```python
from build123d import *

# Parameters (mm, degrees)
SKETCH_1_W               = 362
SKETCH_1_H               = 68
SM_BASE_FLANGE_1_DEPTH   = 1.5
SKETCH_6_R               = 2.5
CUT_EXTRUDE_1_DEPTH      = 10
SKETCH_7_W               = 40
SKETCH_7_H               = 42
SM_BASE_FLANGE_1_2_DEPTH = 1.5
SM_EDGE_FLANGE_1_DEPTH   = 422


# Sheet-metal steps are written as plain solids
with BuildPart() as part:
    # Sketch 1 → Sm Base Flange 1 (new body)
    with BuildSketch(Plane(origin=(0, 0, 0), x_dir=(0, 0, -1), z_dir=(1, 0, 0))):
        with Locations((0, -34)):
            Rectangle(SKETCH_1_W, SKETCH_1_H)
    extrude(amount=-SM_BASE_FLANGE_1_DEPTH)

    # Эскиз6 → Вырез-Вытянуть1 (cut)
    with BuildSketch(Plane(origin=(0, 0, 0), x_dir=(0, 0, -1), z_dir=(1, 0, 0))):
        with Locations((158, -10)):
            Circle(SKETCH_6_R)
        with Locations((128, -10)):
            Circle(SKETCH_6_R)
        with Locations(Location((-128, -10, 0), (0, 0, 180))):
            Circle(SKETCH_6_R)
        with Locations(Location((-158, -10, 0), (0, 0, 180))):
            Circle(SKETCH_6_R)
    extrude(amount=-CUT_EXTRUDE_1_DEPTH, mode=Mode.SUBTRACT)

    # Эскиз7 → Sm Base Flange 1 2 (add)
    with BuildSketch(Plane(origin=(0, 0, 0), x_dir=(0, 0, -1), z_dir=(1, 0, 0))):
        with Locations((-201, -21)):
            Rectangle(SKETCH_7_W, SKETCH_7_H)
        with Locations((201, -21)):
            Rectangle(SKETCH_7_W, SKETCH_7_H)
    extrude(amount=-SM_BASE_FLANGE_1_2_DEPTH)

    # Ребро-кромка1 section (across the edge) → Ребро-кромка1 (add)
    with BuildSketch(Plane(origin=(0, 1.5, -211), x_dir=(0, -1, 0), z_dir=(0, 0, 1))):
        with BuildLine():
            Line((-1.5, 1.5), (-1.5, 12))
            Line((-1.5, 12), (0, 12))
            Line((0, 12), (0, 1.5))
            ThreePointArc((0, 1.5), (0.439339828, 0.439339828), (1.5, 0))
            Line((1.5, 0), (1.5, -1.5))
            ThreePointArc((1.5, -1.5), (-0.621320344, -0.621320344), (-1.5, 1.5))
        make_face()
    extrude(amount=SM_EDGE_FLANGE_1_DEPTH)


solid = part.part
```
Verification items for the finished model (mm, model axes). A direction names the side the tool comes from. Give positions to 0.01 mm unless a question says otherwise; leave off trailing zeros. Loops run counter-clockwise (first coordinate to the right, second up) from the corner with the lowest first, then second, coordinate; pieces in that order, holes last. Notation, with made-up numbers: M 41,14 L 84,14 A7 ccw 84,24 Z; hole C -21,-39.5 d3. An arc over 180 degrees is marked long. One line per question, with ' | ' between items.
Item 1: Section check B-B, the plane y = -46.5. Record the cut outline in (x, z), plus the area to 3 significant figures.
Completed:
outline: M -1.5,-181 L 0,-181 L 0,181 L -1.5,181 Z | area: 543 mm^2
Item 2: Thickness scan on line 1 (Y direction, x = -1.05, z = -158); line 2 (X direction, y = -7, z = -16); line 3 (Y direction, x = 8.5, z = 94). Record the ranges inside material, lowest first. Write a range as [from, to].
Completed:
line 1: y = [-68, -12.5], [-7.5, 1.58] | line 2: x = [-1.5, 0] | line 3: y = [1.5, 3]
Item 3: Depth check by flat-ended pin: P1, Ø0.8, axis at x = -1, z = 214, coming from the +Y side; P2, Ø1.6, axis at x = -0.5, z = -195.5, coming from the -Y side; P3, Ø8, axis at x = 3.5, y = -59, coming from the -Z side; P4, Ø0.9, axis at x = 2, y = 1, coming from the -Z side. Enter the tip coordinate at first touch or a pass-through.
Completed:
P1: stops at y = 0 | P2: stops at y = -42 | P3: stops at z = -181 | P4: passes through
Item 4: Section check A-A, the plane z = -104. Record the cut outline in (x, y).
Completed:
outline: M -1.5,-68 L 0,-68 L 0,0 A1.5 cw 1.5,1.5 L 12,1.5 L 12,3 L 1.5,3 A3 ccw -1.5,0 Z
Item 5: Tool access check on faces 1 (the face through (7, 1.5, -3)), 2 (the face through (-1.5, -34, 3)). Record the directions out of +Z, -Z, +X, -X, +Y, -Y that give a thin tool (end or side, any length) a straight path to the whole face; none if there is none.
Completed:
face 1: +Z, -Z, +X, -Y | face 2: +Z, -Z, -X, +Y, -Y
Item 6: Section check C-C, the plane x = 7. Record the cut outline in (y, z), plus the area to 3 significant figures.
Completed:
outline: M 1.5,-211 L 3,-211 L 3,211 L 1.5,211 Z | area: 633 mm^2
